```python
from build123d import *

# Parameters (mm, degrees)
F1_DEPTH       = 1993.9
F2_W           = 152.4
F2_H           = 152.4
F3_DEPTH       = 12.7
F5_D           = 13.49248
F5_CSINK_D     = 23.8252
F5_CSINK_ANGLE = 82


with BuildPart() as f1:
    # F0 (on Front) → F1 (new body)
    with BuildSketch(Plane.XZ):
        Polygon((0, 12.7), (0, 0), (152.4, 0), (152.4, 12.7), (101.6, 12.7), (114.3, 25.4), (38.1, 25.4), (50.8, 12.7), align=None)
    extrude(amount=F1_DEPTH)

    # F2 (on face) → F3 (cut, through all)
    with BuildSketch(Plane.XY.offset(25.4)):
        with Locations((76.2, -76.2)):
            Rectangle(F2_W, F2_H)
        with Locations((76.2, -1917.7)):
            Rectangle(F2_W, F2_H)
    extrude(amount=-F3_DEPTH, mode=Mode.SUBTRACT)

    # F5 (through all)
    with Locations(Plane.XY.offset(12.7)):
        with Locations((38.1, -50.8), (114.3, -50.8), (38.1, -1943.1), (114.3, -1943.1)):
            CounterSinkHole(F5_D / 2, F5_CSINK_D / 2, counter_sink_angle=F5_CSINK_ANGLE)


solid = f1.part
```
CAD build for the part. Positions are in the model's coordinates, mm. Coordinates: 2 decimals unless noted, no trailing zeros. Order: outer loops, then holes, each group sorted by start corner. A loop starts at its lowest first (then second) coordinate and runs counter-clockwise, first axis right, second up. Notation, with made-up numbers: (44, 80) -> (85, 80) arc R15 cw to (85, 98) -> close; hole circle Ø2 at (-4, 80.5). An arc over 180 degrees is marked (long way). Use one line per item in the form item = value. Start each with the question number.
1) Drop flat-ended pins along their axis: pin 1 (4 mm diameter, centred on x = 66, z = 20.5, fed in from +Y); pin 2 (12 mm diameter, centred on x = 114.3, y = -50.8, fed in from -Z); pin 3 (4 mm diameter, centred on x = 67.5, z = 18.5, fed in from -Y). Give the stop position or say it passes through.
2) Band-saw the part on C-C on z = 17.75. Give the cut face in (x, y), then the cut area to 3 significant figures.
3) Pull direction Z, two halves, no side cores. Call faces 1 (the flat face through (111, -983, 12.7)), 2 (the flat face through (75, -983, 0)), 3 (the flat face through (77, -985, 25.4)): +Z half, -Z half, draft (parallel to the pull), parting line (faces both ways), or undercut.
4) Drill centre lines: L1, parallel to Y at x = 38.1, z = 4.5; L2, parallel to X at y = -50.8, z = 4; L3, parallel to Y at x = 65.5, z = 22.5. Where is each one in solid material? Low to high. Write a range as [from, to].
5) Band-saw the part on A-A on y = -997. Give the cut face in (x, z), then the cut area to 3 significant figures.
6) Band-saw the part on B-B on x = 83. Give the cut face in (y, z).
Entries:
q1.pin_1 = -152.4
q1.pin_2 = through
q1.pin_3 = -1841.5
q2.outline = (45.75, -1841.5) -> (106.65, -1841.5) -> (106.65, -152.4) -> (45.75, -152.4) -> close
q2.area = 103,000 mm2
q3.face_1 = undercut
q3.face_2 = -Z half
q3.face_3 = +Z half
q4.L1 = [-1993.9, -1949.85], [-1936.35, -57.55], [-44.05, 0]
q4.L2 = [0, 31.35], [44.85, 107.55], [121.05, 152.4]
q4.L3 = [-1841.5, -152.4]
q5.outline = (0, 0) -> (152.4, 0) -> (152.4, 12.7) -> (101.6, 12.7) -> (114.3, 25.4) -> (38.1, 25.4) -> (50.8, 12.7) -> (0, 12.7) -> close
q5.area = 2,740 mm2
q6.outline = (-1993.9, 0) -> (0, 0) -> (0, 12.7) -> (-152.4, 12.7) -> (-152.4, 25.4) -> (-1841.5, 25.4) -> (-1841.5, 12.7) -> (-1993.9, 12.7) -> close
